from build123d import *

# Parameters (mm, degrees)
BOSS_EXTRUDE1_DEPTH    = 2.54
F_10_CLEARANCE_HOLE1_D = 5.1054


with BuildPart() as part:
    # Sketch1 → Boss-Extrude1 (new body)
    with BuildSketch(Plane.XY):
        Polygon((0, 0), (241.3, 0), (241.3, 203.2), (114.3, 203.2), align=None)
    extrude(amount=BOSS_EXTRUDE1_DEPTH)

    # #10 Clearance Hole1 (through all)
    with Locations(Plane.XY.offset(2.54)):
        with Locations((203.2, 152.4), (228.6, 127), (203.2, 127), (228.6, 152.4)):
            Hole(F_10_CLEARANCE_HOLE1_D / 2)


solid = part.part
For this review, take the finished solid that the model builds, in its own axes (mm). Round coordinates to 2 decimals unless told otherwise and drop trailing zeros. Write each loop counter-clockwise with the first axis right and the second up, starting at its lowest first coordinate (ties: lowest second). Pieces come first, ordered by that corner, then holes. Notation, with made-up numbers: (17.25, -1) -> (48.25, -1) arc R25 cw to (48.25, 36) -> close; hole circle Ø4 at (73, -20.5). An arc over 180 degrees is marked (long way). Use CSV: the item, a comma, the result in double quotes.
(1) Clearance check with flat-ended pins moving along their axes: P1, Ø4.5, axis at x = 203.2, y = 152.4, coming from the -Z side; P2, Ø1.5, axis at x = 80, z = 1, coming from the +Y side; P3, Ø1.5, axis at y = 155, z = 1, coming from the -X side. State where each tip first meets the part, or that it passes through.
Computed values:
P1,"through"
P2,"y = 143.56"
P3,"x = 86.77"
(2) Consider section C-C, the plane y = 152.4. Give the boundary of the cut face in (x, z) (3 decimals), plus the area to 3 significant figures.
Computed values:
outline,"(85.725, 0) -> (200.647, 0) -> (200.647, 2.54) -> (85.725, 2.54) -> close; (205.753, 0) -> (226.047, 0) -> (226.047, 2.54) -> (205.753, 2.54) -> close; (231.153, 0) -> (241.3, 0) -> (241.3, 2.54) -> (231.153, 2.54) -> close"
area,"369 mm²"
(3) Consider section A-A, the plane z = 1.9. Give the boundary of the cut face in (x, y).
Computed values:
outline,"(0, 0) -> (241.3, 0) -> (241.3, 203.2) -> (114.3, 203.2) -> close; hole circle Ø5.11 at (203.2, 127); hole circle Ø5.11 at (203.2, 152.4); hole circle Ø5.11 at (228.6, 127); hole circle Ø5.11 at (228.6, 152.4)"
(4) Draft analysis for pull direction Y (two halves, no side actions). For faces 1 (the face through (146, 103, 0)), 2 (the face through (227.422, 150.135, 1.252)), 3 (the face through (57.95, 103.02, 1.25)), state which applies: +Y half, -Y half, draft (parallel to the pull), parting line (faces both ways), or undercut.
Computed values:
face 1,"draft"
face 2,"undercut"
face 3,"+Y half"
(5) To check wall thickness, follow L1, parallel to Y at x = 203.2, z = 1.15; L2, parallel to X at y = 152.4, z = 1.2 (3 decimals); L3, parallel to X at y = 103, z = 0.65. State the ranges of each line that lie inside material, in increasing order. Write a range as [from, to].
Computed values:
L1,"[0, 124.45], [129.55, 149.85], [154.95, 203.2]"
L2,"[85.725, 200.647], [205.753, 226.047], [231.153, 241.3]"
L3,"[57.94, 241.3]"
(6) Consider section D-D, the plane x = 18. Give the boundary of the cut face in (y, z).
Computed values:
outline,"(0, 0) -> (32, 0) -> (32, 2.54) -> (0, 2.54) -> close"
(7) Consider section B-B, the plane x = 203.2. Give the boundary of the cut face in (y, z).
Computed values:
outline,"(0, 0) -> (124.45, 0) -> (124.45, 2.54) -> (0, 2.54) -> close; (129.55, 0) -> (149.85, 0) -> (149.85, 2.54) -> (129.55, 2.54) -> close; (154.95, 0) -> (203.2, 0) -> (203.2, 2.54) -> (154.95, 2.54) -> close"
